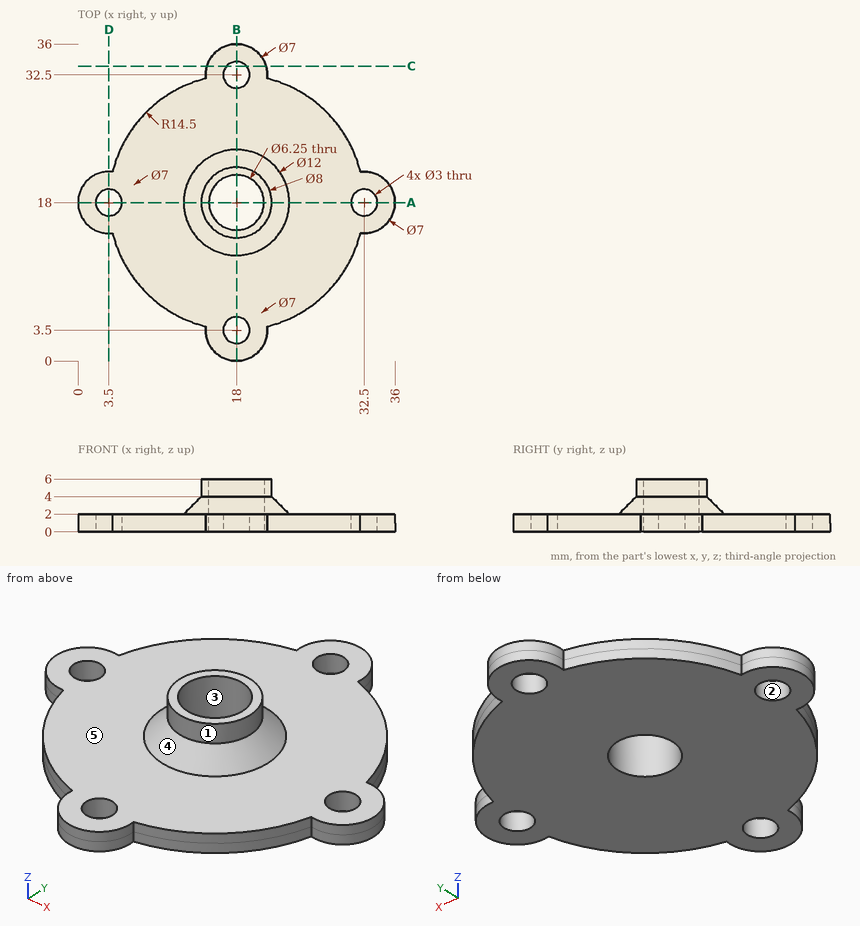
Study the drawing (mm; zero at the part's minimum x, y, z) and answer. A direction names the side the tool comes from. Coordinates: 2 decimals unless noted, no trailing zeros. Loops run counter-clockwise (first coordinate to the right, second up) from the corner with the lowest first, then second, coordinate; pieces in that order, holes last. Notation, with made-up numbers: M 3,83.5 L 47,83.5 A34 ccw 47,120.5 Z; hole C 74,75.25 d2. An arc over 180 degrees is marked long. Answer in a Markdown table with one row per item.
1) Which of the six approach directions +Z, -Z, +X, -X, +Y, -Y give full straight-line access (tool end or side, diameter ignored) to the marked faces 1 and 2?
Answers below:
| item | result |
|---|---|
| face 1 | +Z |
| face 2 | +Z, -Z |
2) Find section A-A (y = 18). Determine the outline of the cut face in (x, z) (3 decimals), then the cut area to 3 significant figures.
Answers below:
| item | result |
|---|---|
| outline | M 0,0 L 2,0 L 2,2 L 0,2 Z; M 5,0 L 14.875,0 L 14.875,6 L 14,6 L 14,4 L 12,2 L 5,2 Z; M 21.125,0 L 31,0 L 31,2 L 24,2 L 22,4 L 22,6 L 21.125,6 Z; M 34,0 L 36,0 L 36,2 L 34,2 Z |
| area | 58.5 mm^2 |
3) Find the intervals of material crossed by probe 1 along Y at (x, z) = (18, 1.7) (3 decimals); probe 2 along Y at (x, z) = (18, 4.3) (3 decimals); probe 3 along Y at (x, z) = (32.5, 1.3), in increasing order.
Answers below:
| item | result |
|---|---|
| probe 1 | 0 to 2, 5 to 14.875, 21.125 to 31, 34 to 36 |
| probe 2 | 14 to 14.875, 21.125 to 22 |
| probe 3 | 14.5 to 16.5, 19.5 to 21.5 |
4) Determine the mould class of the marked faces 3, 4 and 5 for opening direction X: released by +X, released by -X, zero draft, split by the parting line, or undercut.
Answers below:
| item | result |
|---|---|
| face 3 | undercut |
| face 4 | split by the parting line |
| face 5 | zero draft |
5) Find section D-D (x = 3.5). Determine the outline of the cut face in (y, z), then the cut area to 3 significant figures.
Answers below:
| item | result |
|---|---|
| outline | M 14.5,0 L 16.5,0 L 16.5,2 L 14.5,2 Z; M 19.5,0 L 21.5,0 L 21.5,2 L 19.5,2 Z |
| area | 8.00 mm^2 |
6) Find section C-C (y = 33.5). Determine the outline of the cut face in (x, z).
Answers below:
| item | result |
|---|---|
| outline | M 14.65,0 L 16.88,0 L 16.88,2 L 14.65,2 Z; M 19.12,0 L 21.35,0 L 21.35,2 L 19.12,2 Z |
